Can you work these out from the model? Positions are in its coordinate system, mm. A direction names the side the tool comes from. Give positions to 0.01 mm unless a question says otherwise; leave off trailing zeros. Write each loop counter-clockwise with the first axis right and the second up, starting at its lowest first coordinate (ties: lowest second). Pieces come first, ordered by that corner, then holes. Notation, with made-up numbers: (78.25, -38.75) - (90.25, -38.75) arc R7 cw to (90.25, -31.75) - close; hole circle Ø7 at (36.25, -25). An arc over 180 degrees is marked (long way). Use a Markdown table: item, result. Add a question column.
```python
from build123d import *

# Parameters (mm, degrees)
SKETCH_1_W          = 27.7
SKETCH_1_H          = 27.7
EXTRUDE_1_DEPTH     = 70
SKETCH_2_R          = 2.075
CUT_EXTRUDE_1_DEPTH = 70
CUT_EXTRUDE_2_DEPTH = 70
FILLET_1_R          = 3


with BuildPart() as part:
    # 草图1 → 凸台-拉伸1 (new body)
    with BuildSketch(Plane(origin=(0, 0, 0), x_dir=(1, 0, 0), z_dir=(0, 1, 0))):
        Rectangle(SKETCH_1_W, SKETCH_1_H)
    extrude(amount=EXTRUDE_1_DEPTH)

    # 草图2 → 切除-拉伸1 (cut)
    with BuildSketch(Plane.XY.offset(13.85)):
        with Locations((0, 4)):
            Circle(SKETCH_2_R)
        with Locations((0, 30.5)):
            Circle(SKETCH_2_R)
        with Locations((0, 61.5)):
            Circle(SKETCH_2_R)
    extrude(amount=-CUT_EXTRUDE_1_DEPTH, mode=Mode.SUBTRACT)

    # 草图3 → 切除-拉伸2 (cut)
    with BuildSketch(Plane.ZY.offset(13.85)):
        with BuildLine():
            Line((-8, 25), (-8, 45))
            ThreePointArc((-8, 45), (0, 53), (8, 45))
            Line((8, 45), (8, 25))
            ThreePointArc((8, 25), (0, 17), (-8, 25))
        make_face()
    extrude(amount=-CUT_EXTRUDE_2_DEPTH, mode=Mode.SUBTRACT)

    # 圆角1
    fillet_1_edges = [part.edges().sort_by_distance(p)[0] for p in [
        (13.85, 35, 13.85),
        (-13.85, 35, 13.85),
        (-13.85, 35, -13.85),
        (13.85, 35, -13.85),
    ]]
    fillet(fillet_1_edges, radius=FILLET_1_R)


solid = part.part
```
Q1. If we mould it in two halves opening along Y, with no side actions, what happens to faces 3 (the cylindrical face through (-12.99, 35.49, 12.95)), 4 (the flat face through (0, 35, 8)), 5 (the flat face through (0, 0, 0))? For each: released by +Y, released by -Y, zero draft, split by the parting line, or undercut.
Q2. Suppose I cut it at A-A (z = 0). Please give me the cut outline in (x, y) (3 decimals).
Q3. I'm going to push a flat-ended pin straight in: P1, Ø4, axis at x = 4.5, z = 10, coming from the -Y side. Where does the tip first touch, or does it pass through?
Q4. If I drill on probe 1 along Y at (x, z) = (0, 12.3) (3 decimals); probe 2 along Z at (x, y) = (-5.75, 28.5); probe 3 along Y at (x, z) = (0, 3.75) (3 decimals), over which ranges is the centre line in solid material (lowest first)? Write a range as [from, to].
Q5. Suppose I cut it at B-B (x = 0). Please give me the cut outline in (y, z) (3 decimals).
Q6. On a 3-axis mill with a long thin cutter (end or side, diameter ignored), from which of +Z, -Z, +X, -X, +Y, -Y can I reach the whole of each face in a straight line? I mean faces 1 (the flat face through (0, 35, -13.85)), 2 (the cylindrical face through (0, 53, 0)). Say none if no direction works.
Q7. Suppose I cut it at D-D (y = 4). Please give me the cut outline in (x, z) (3 decimals).
Q8. Suppose I cut it at C-C (y = 30.5). Please give me the cut outline in (x, z) (3 decimals), and give its area (3 significant figures).
Derived:
| question | item | result |
|---|---|---|
| 1 | face 3 | zero draft |
| 1 | face 4 | undercut |
| 1 | face 5 | released by -Y |
| 2 | outline | (-13.85, 0) - (13.85, 0) - (13.85, 17) - (-13.85, 17) - close; (-13.85, 53) - (13.85, 53) - (13.85, 70) - (-13.85, 70) - close; hole circle Ø4.15 at (0, 4); hole circle Ø4.15 at (0, 61.5) |
| 3 | P1 | y = 0 |
| 4 | probe 1 | [0, 1.925], [6.075, 28.425], [32.575, 59.425], [63.575, 70] |
| 4 | probe 2 | [-13.85, -8], [8, 13.85] |
| 4 | probe 3 | [0, 1.925], [6.075, 17.933], [52.067, 59.425], [63.575, 70] |
| 5 | outline | (0, -13.85) - (1.925, -13.85) - (1.925, 13.85) - (0, 13.85) - close; (6.075, -13.85) - (28.425, -13.85) - (28.425, -8) - (25, -8) arc R8 cw to (25, 8) - (28.425, 8) - (28.425, 13.85) - (6.075, 13.85) - close; (32.575, -13.85) - (59.425, -13.85) - (59.425, 13.85) - (32.575, 13.85) - (32.575, 8) - (45, 8) arc R8 cw to (45, -8) - (32.575, -8) - close; (63.575, -13.85) - (70, -13.85) - (70, 13.85) - (63.575, 13.85) - close |
| 6 | face 1 | -Z, +X, -X, +Y, -Y |
| 6 | face 2 | +X, -X |
| 7 | outline | (-13.85, -10.85) arc R3 ccw to (-10.85, -13.85) - (-2.075, -13.85) - (-2.075, 13.85) - (-10.85, 13.85) arc R3 ccw to (-13.85, 10.85) - close; (2.075, -13.85) - (10.85, -13.85) arc R3 ccw to (13.85, -10.85) - (13.85, 10.85) arc R3 ccw to (10.85, 13.85) - (2.075, 13.85) - close |
| 8 | outline | (-13.85, -10.85) arc R3 ccw to (-10.85, -13.85) - (-2.075, -13.85) - (-2.075, -8) - (-13.85, -8) - close; (-13.85, 8) - (-2.075, 8) - (-2.075, 13.85) - (-10.85, 13.85) arc R3 ccw to (-13.85, 10.85) - close; (2.075, -13.85) - (10.85, -13.85) arc R3 ccw to (13.85, -10.85) - (13.85, -8) - (2.075, -8) - close; (2.075, 8) - (13.85, 8) - (13.85, 10.85) arc R3 ccw to (10.85, 13.85) - (2.075, 13.85) - close |
| 8 | area | 268 mm² |
